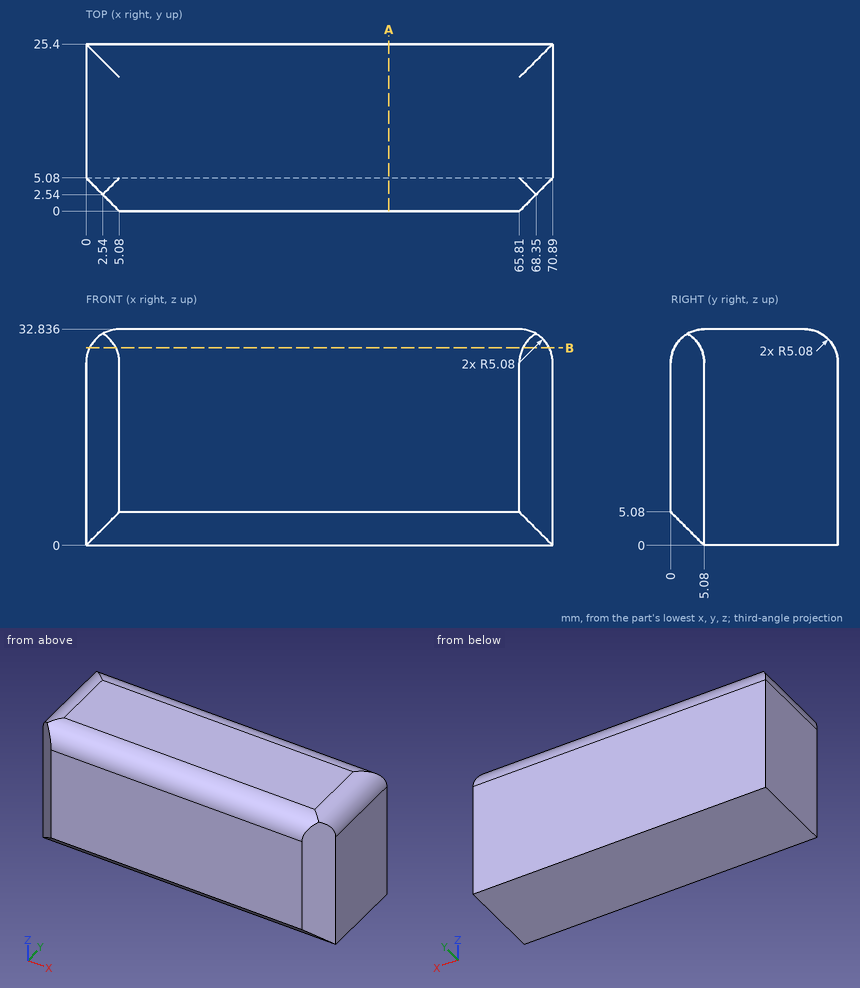
Job drawing, mm, ordinate dimensions from the low corner. One solid piece. Coordinates: 2 decimals unless noted, no trailing zeros. Order: outer loops, then holes, each group sorted by start corner. A loop starts at its lowest first (then second) coordinate and runs counter-clockwise, first axis right, second up. Notation, with made-up numbers: (-8.5, 6) - (42.5, 6) arc R16 cw to (42.5, 21) - close; hole circle Ø9 at (34, 76.5). An arc over 180 degrees is marked (long way). Write each question's results on one line, items separated by ' | '. Start each with the question number.
Item 1: Band-saw the part on B-B on z = 30. Write the cut outline in (x, y), and give its area (3 significant figures).
Item 2: Wall check: probe 1 along X at (y, z) = (6.5, 28) (1 decimal); probe 2 along Y at (x, z) = (46, 28) (1 decimal); probe 3 along Z at (x, y) = (45.5, 4.25). Give the ranges that are in metal, low to high. Write a range as [from, to].
Item 3: Band-saw the part on A-A on x = 46. Write the cut outline in (y, z), and give its area (3 significant figures).
Numbers:
1) outline: (0.52, 4.56) - (4.56, 0.52) - (66.33, 0.52) - (70.37, 4.56) - (70.37, 24.88) - (0.52, 24.88) - close | area: 1,680 mm^2
2) probe 1: [0, 70.9] | probe 2: [0, 25.4] | probe 3: [0.83, 32.77]
3) outline: (0, 5.08) - (5.08, 0) - (25.4, 0) - (25.4, 27.76) arc R5.08 ccw to (20.32, 32.84) - (5.08, 32.84) arc R5.08 ccw to (0, 27.76) - close | area: 810 mm^2
